Build history of the part. All positions in model axes, mm. A direction names the side the tool comes from. Coordinates: 2 decimals unless noted, no trailing zeros. Loops run counter-clockwise (first coordinate to the right, second up) from the corner with the lowest first, then second, coordinate; pieces in that order, holes last. Notation, with made-up numbers: (48, -3.75) -> (76, -3.75) arc R18 cw to (76, 15.25) -> close; hole circle Ø10 at (89, -34). An arc over 180 degrees is marked (long way). One line per item, written item: value. Start each with the question number.
```python
from build123d import *

# Parameters (mm, degrees)
SKETCH2_W                                       = 74
SKETCH2_H                                       = 10
BOSS_EXTRUDE1_DEPTH                             = 2.5
SKETCH3_W                                       = 2.5
SKETCH3_H                                       = 10
BOSS_EXTRUDE2_DEPTH                             = 10
CSK_FOR_M2_FLAT_HEAD_MACHINE_SCREW1_D           = 2.4
CSK_FOR_M2_FLAT_HEAD_MACHINE_SCREW1_DEPTH       = 2.5
CSK_FOR_M2_FLAT_HEAD_MACHINE_SCREW1_CSINK_D     = 4.4
CSK_FOR_M2_FLAT_HEAD_MACHINE_SCREW1_CSINK_ANGLE = 90
CSK_FOR_M2_FLAT_HEAD_MACHINE_SCREW2_D           = 2.4
CSK_FOR_M2_FLAT_HEAD_MACHINE_SCREW2_DEPTH       = 2.5
CSK_FOR_M2_FLAT_HEAD_MACHINE_SCREW2_CSINK_D     = 4.4
CSK_FOR_M2_FLAT_HEAD_MACHINE_SCREW2_CSINK_ANGLE = 90


with BuildPart() as part:
    # Sketch2 → Boss-Extrude1 (new body)
    with BuildSketch(Plane(origin=(0, 0, 0), x_dir=(1, 0, 0), z_dir=(0, 1, 0))):
        with Locations((25.358263924, 0.691988738)):
            Rectangle(SKETCH2_W, SKETCH2_H)
    extrude(amount=BOSS_EXTRUDE1_DEPTH)

    # Sketch3 → Boss-Extrude2 (add)
    with BuildSketch(Plane(origin=(0, 2.5, 0), x_dir=(1, 0, 0), z_dir=(0, 1, 0))):
        with Locations((-10.391736076, 0.691988738)):
            Rectangle(SKETCH3_W, SKETCH3_H)
        with Locations((61.108263924, 0.691988738)):
            Rectangle(SKETCH3_W, SKETCH3_H)
    extrude(amount=BOSS_EXTRUDE2_DEPTH)

    # CSK for M2 Flat Head Machine Screw1
    with Locations(Plane.ZY.offset(-59.858263924)):
        with Locations((-0.691988738, 7.5)):
            CounterSinkHole(CSK_FOR_M2_FLAT_HEAD_MACHINE_SCREW1_D / 2, CSK_FOR_M2_FLAT_HEAD_MACHINE_SCREW1_CSINK_D / 2, depth=CSK_FOR_M2_FLAT_HEAD_MACHINE_SCREW1_DEPTH, counter_sink_angle=CSK_FOR_M2_FLAT_HEAD_MACHINE_SCREW1_CSINK_ANGLE)

    # CSK for M2 Flat Head Machine Screw2
    with Locations(Plane(origin=(-9.141736076, 0, 0), x_dir=(0, 0, -1), z_dir=(1, 0, 0))):
        with Locations((0.691988738, 7.5)):
            CounterSinkHole(CSK_FOR_M2_FLAT_HEAD_MACHINE_SCREW2_D / 2, CSK_FOR_M2_FLAT_HEAD_MACHINE_SCREW2_CSINK_D / 2, depth=CSK_FOR_M2_FLAT_HEAD_MACHINE_SCREW2_DEPTH, counter_sink_angle=CSK_FOR_M2_FLAT_HEAD_MACHINE_SCREW2_CSINK_ANGLE)


solid = part.part
```
Item 1: Two-plate mould, pull along X, no slides. Class faces 3 (the face through (-9.142, 7, 2)), 4 (the face through (-10.9, 8.69, -0.85)), 5 (the face through (-11.642, 6, -1)), 6 (the face through (62.358, 6, -1)): +X half, -X half, draft (parallel to the pull), parting line (faces both ways), or undercut.
Item 2: Band-saw the part on A-A, the plane y = 7.5. List the corners of the cut face in (x, z), and give its area (3 significant figures).
Item 3: Band-saw the part on C-C, the plane z = -4.75. List the corners of the cut face in (x, y), and give its area (3 significant figures).
Item 4: Band-saw the part on B-B, the plane y = 11.5. List the corners of the cut face in (x, z).
Item 5: Band-saw the part on D-D, the plane x = 12. List the corners of the cut face in (y, z).
Item 6: Tool access for faces 1 (the face through (59.858, 7, 2)), 2 (the face through (25, 2, -5.692)): list every direction of +Z, -Z, +X, -X, +Y, -Y with a clear straight run to the whole face (end or side of a thin tool).
Item 7: Probe probe 1 along X at (y, z) = (8, -4); probe 2 along Z at (x, y) = (61.4, 7.5); probe 3 along Y at (x, z) = (1.5, -3). List the from-to ranges inside material, lowest first.
Item 8: Drop a flat-ended pin along its axis: pin 1 Ø3 at (y, z) = (7.5, -0.69) entering from +X. Give the stop position or say it passes through.
Worked out:
1. face 3: undercut
1. face 4: draft
1. face 5: -X half
1. face 6: +X half
2. outline: (-11.64, -5.69) -> (-9.14, -5.69) -> (-9.14, -2.89) -> (-10.14, -1.89) -> (-11.64, -1.89) -> close; (-11.64, 0.51) -> (-10.14, 0.51) -> (-9.14, 1.51) -> (-9.14, 4.31) -> (-11.64, 4.31) -> close; (59.86, -5.69) -> (62.36, -5.69) -> (62.36, -1.89) -> (60.86, -1.89) -> (59.86, -2.89) -> close; (59.86, 1.51) -> (60.86, 0.51) -> (62.36, 0.51) -> (62.36, 4.31) -> (59.86, 4.31) -> close
2. area: 36.0 mm²
3. outline: (-11.64, 0) -> (62.36, 0) -> (62.36, 12.5) -> (59.86, 12.5) -> (59.86, 2.5) -> (-9.14, 2.5) -> (-9.14, 12.5) -> (-11.64, 12.5) -> close
3. area: 235 mm²
4. outline: (-11.64, -5.69) -> (-9.14, -5.69) -> (-9.14, 4.31) -> (-11.64, 4.31) -> close; (59.86, -5.69) -> (62.36, -5.69) -> (62.36, 4.31) -> (59.86, 4.31) -> close
5. outline: (0, -5.69) -> (2.5, -5.69) -> (2.5, 4.31) -> (0, 4.31) -> close
6. face 1: +Z, -Z, +Y
6. face 2: -Z, +X, -X, +Y, -Y
7. probe 1: x = -11.64 to -9.14, 59.86 to 62.36
7. probe 2: z = -5.69 to -1.89, 0.51 to 4.31
7. probe 3: y = 0 to 2.5
8. pin 1: stops at x = 62.36
